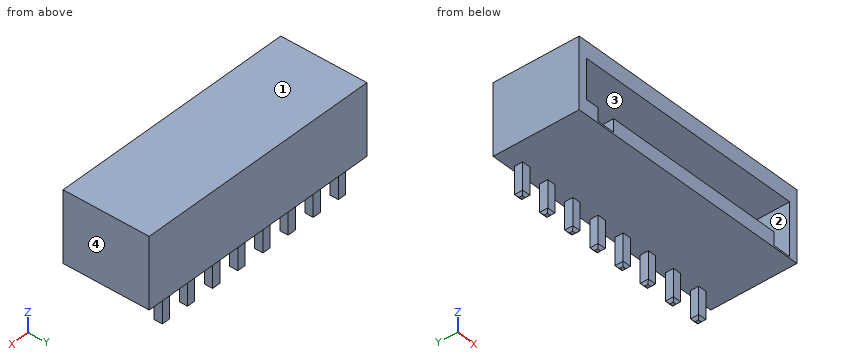
from build123d import *

# Parameters (mm, degrees)
SKETCH_1_W                         = 30.3
SKETCH_1_H                         = 10.5
EXTRUDE_1_DEPTH                    = 8.6
CUT_EXTRUDE_1_DEPTH                = 7
EXTRUDE_START                      = -5
SKETCH_3_W                         = 1
SKETCH_3_H                         = 1
EXTRUDE_2_DEPTH                    = 8.6
CHAMFER_1_SIZE                     = 0.3
PATTERN_LINEAR_1_COUNT             = 8
PATTERN_LINEAR_1_PITCH             = 3.5
CHAMFER_1_OF_PATTERN_LINEAR_1_SIZE = 0.3


with BuildPart() as part:
    # Эскиз1 → Бобышка-Вытянуть1 (new body)
    with BuildSketch(Plane.XY):
        Rectangle(SKETCH_1_W, SKETCH_1_H)
    extrude(amount=EXTRUDE_1_DEPTH)

    # Эскиз2 → Вырез-Вытянуть1 (cut)
    with BuildSketch(Plane.XZ.offset(5.25)):
        Polygon((-14.15, 6.6), (14.15, 6.6), (14.15, 0.2), (11.95, 0.2), (11.95, 1.8), (-10.35, 1.8), (-10.35, 0.2), (-12.55, 0.2), (-12.55, 1.8), (-14.15, 1.8), align=None)
    extrude(amount=-CUT_EXTRUDE_1_DEPTH, mode=Mode.SUBTRACT)

    # Эскиз3 → Бобышка-Вытянуть2 (add)
    with BuildSketch(Plane(origin=(0, 0, 0), x_dir=(-1, 0, 0), z_dir=(0, 0, -1)).offset(EXTRUDE_START)):
        with Locations((12.25, 4.25)):
            Rectangle(SKETCH_3_W, SKETCH_3_H)
    extrude_2 = extrude(amount=EXTRUDE_2_DEPTH)

    # Фаска1
    chamfer_1_edges = [part.edges().sort_by_distance(p)[0] for p in [
        (-11.75, 4.25, -3.6),
        (-12.25, 3.75, -3.6),
        (-12.75, 4.25, -3.6),
        (-12.25, 4.75, -3.6),
    ]]
    chamfer(chamfer_1_edges, length=CHAMFER_1_SIZE)

    # Линейный массив1: Бобышка-Вытянуть2 ×8
    with Locations(*[(i * PATTERN_LINEAR_1_PITCH, 0, 0) for i in range(1, PATTERN_LINEAR_1_COUNT)]):
        add(extrude_2)

    # Фаска1 of Линейный массив1
    chamfer_1_of_pattern_linear_1_edges = [part.edges().sort_by_distance(p)[0] for p in [
        (-8.25, 4.25, -3.6),
        (-8.75, 3.75, -3.6),
        (-9.25, 4.25, -3.6),
        (-8.75, 4.75, -3.6),
        (-4.75, 4.25, -3.6),
        (-5.25, 3.75, -3.6),
        (-5.75, 4.25, -3.6),
        (-5.25, 4.75, -3.6),
        (-1.25, 4.25, -3.6),
        (-1.75, 3.75, -3.6),
        (-2.25, 4.25, -3.6),
        (-1.75, 4.75, -3.6),
        (2.25, 4.25, -3.6),
        (1.75, 3.75, -3.6),
        (1.25, 4.25, -3.6),
        (1.75, 4.75, -3.6),
        (5.75, 4.25, -3.6),
        (5.25, 3.75, -3.6),
        (4.75, 4.25, -3.6),
        (5.25, 4.75, -3.6),
        (9.25, 4.25, -3.6),
        (8.75, 3.75, -3.6),
        (8.25, 4.25, -3.6),
        (8.75, 4.75, -3.6),
        (12.75, 4.25, -3.6),
        (12.25, 3.75, -3.6),
        (11.75, 4.25, -3.6),
        (12.25, 4.75, -3.6),
    ]]
    chamfer(chamfer_1_of_pattern_linear_1_edges, length=CHAMFER_1_OF_PATTERN_LINEAR_1_SIZE)


solid = part.part
Design review of the part built by this model. Coordinates are the model's own, in mm. Face numbers are marked on the shaded views. Coordinates: 2 decimals unless noted, no trailing zeros. Order: outer loops, then holes, each group sorted by start corner. A loop starts at its lowest first (then second) coordinate and runs counter-clockwise, first axis right, second up. Notation, with made-up numbers: (39.5, -27.5) -> (79.5, -27.5) arc R29 cw to (79.5, 4.5) -> close; hole circle Ø9 at (31, 63). An arc over 180 degrees is marked (long way). One line per item, written item: value.
1) Clearance check with flat-ended pins moving along their axes: P1, Ø1.1, axis at x = -8.5, z = -1.5, coming from the -Y side; P2, Ø1.1, axis at y = 4.5, z = -2, coming from the +X side; P3, Ø0.5, axis at y = 4, z = -2, coming from the -X side. State where each tip first meets the part, or that it passes through.
Output values:
P1: stops at y = 3.75
P2: stops at x = 12.75
P3: stops at x = -12.75
2) We need section C-C, the plane z = 5. Give the boundary of the cut face in (x, y).
Output values:
outline: (-15.15, -5.25) -> (-14.15, -5.25) -> (-14.15, 1.75) -> (14.15, 1.75) -> (14.15, -5.25) -> (15.15, -5.25) -> (15.15, 5.25) -> (-15.15, 5.25) -> close
3) We need section B-B, the plane x = 4. Give the boundary of the cut face in (y, z), then the cut area to 3 significant figures.
Output values:
outline: (-5.25, 0) -> (5.25, 0) -> (5.25, 8.6) -> (-5.25, 8.6) -> (-5.25, 6.6) -> (1.75, 6.6) -> (1.75, 1.8) -> (-5.25, 1.8) -> close
area: 56.7 mm2
4) We need section A-A, the plane y = 0.5. Give the boundary of the cut face in (x, z), then the cut area to 3 significant figures.
Output values:
outline: (-15.15, 0) -> (15.15, 0) -> (15.15, 8.6) -> (-15.15, 8.6) -> close; hole (-14.15, 1.8) -> (-12.55, 1.8) -> (-12.55, 0.2) -> (-10.35, 0.2) -> (-10.35, 1.8) -> (11.95, 1.8) -> (11.95, 0.2) -> (14.15, 0.2) -> (14.15, 6.6) -> (-14.15, 6.6) -> close
area: 118 mm2
5) To check wall thickness, follow probe 1 along X at (y, z) = (0.25, 4.75); probe 2 along Z at (x, y) = (3, 1.5); probe 3 along Z at (x, y) = (-12.5, -3). State the ranges of each line that lie inside material, in increasing order. Write a range as [from, to].
Output values:
probe 1: x = [-15.15, -14.15], [14.15, 15.15]
probe 2: z = [0, 1.8], [6.6, 8.6]
probe 3: z = [0, 0.2], [6.6, 8.6]
6) Draft analysis for pull direction X (two halves, no side actions). For the marked faces 1, 2, 3 and 4, state which applies: +X half, -X half, draft (parallel to the pull), parting line (faces both ways), or undercut.
Output values:
face 1: draft
face 2: undercut
face 3: undercut
face 4: +X half
7) We need section D-D, the plane z = 0.5. Give the boundary of the cut face in (x, y).
Output values:
outline: (-15.15, -5.25) -> (-12.55, -5.25) -> (-12.55, 1.75) -> (-10.35, 1.75) -> (-10.35, -5.25) -> (11.95, -5.25) -> (11.95, 1.75) -> (14.15, 1.75) -> (14.15, -5.25) -> (15.15, -5.25) -> (15.15, 5.25) -> (-15.15, 5.25) -> close
